Can you work these out from the model? Positions are in its coordinate system, mm. Face numbers are marked on the shaded views. A direction names the side the tool comes from. Round coordinates to 2 decimals unless told otherwise and drop trailing zeros. Order: outer loops, then holes, each group sorted by start corner. A loop starts at its lowest first (then second) coordinate and runs counter-clockwise, first axis right, second up. Notation, with made-up numbers: (32.5, 17) -> (68.5, 17) arc R28 cw to (68.5, 52) -> close; hole circle Ø3 at (-33, -31). An arc over 180 degrees is marked (long way). One line per item, written item: value.
```python
from build123d import *

# Parameters (mm, degrees)
F1_DEPTH = 25.4
F2_R     = 1.27
F3_R     = 2.286
F4_DEPTH = 7.62


with BuildPart() as f1:
    # F0 (on Top) → F1 (new body)
    with BuildSketch(Plane.XY):
        with BuildLine():
            Line((-44.880287, 2.54), (-3.81, 2.54))
            ThreePointArc((-3.81, 2.54), (-2.911974, 2.911974), (-2.54, 3.81))
            Line((-2.54, 3.81), (-2.54, 10.16))
            Line((-2.54, 10.16), (-15.24, 10.16))
            Line((-15.24, 10.16), (-15.24, 48.768))
            Line((-15.24, 48.768), (-32.180287, 48.768))
            ThreePointArc((-32.180287, 48.768), (-32.40082, 48.748706), (-32.614652, 48.69141))
            Line((-32.614652, 48.69141), (-52.504366, 41.452146))
            ThreePointArc((-52.504366, 41.452146), (-53.110323, 40.987179), (-53.34, 40.258736))
            Line((-53.34, 40.258736), (-53.34, 39.878))
            ThreePointArc((-53.34, 39.878), (-52.968026, 38.979974), (-52.07, 38.608))
            Line((-52.07, 38.608), (-29.21, 38.608))
            ThreePointArc((-29.21, 38.608), (-28.311974, 38.236026), (-27.94, 37.338))
            Line((-27.94, 37.338), (-27.94, 13.97))
            ThreePointArc((-27.94, 13.97), (-28.311974, 13.071974), (-29.21, 12.7))
            Line((-29.21, 12.7), (-64.77, 12.7))
            ThreePointArc((-64.77, 12.7), (-65.668026, 12.328026), (-66.04, 11.43))
            Line((-66.04, 11.43), (-66.04, 11.049264))
            ThreePointArc((-66.04, 11.049264), (-65.810323, 10.320821), (-65.204366, 9.855854))
            Line((-65.204366, 9.855854), (-45.314652, 2.61659))
            ThreePointArc((-45.314652, 2.61659), (-45.10082, 2.559294), (-44.880287, 2.54))
        make_face()
    extrude(amount=F1_DEPTH)

    # F2
    f2_edges = [f1.edges().sort_by_distance(p)[0] for p in [
        (-15.24, 10.16, 12.7),
        (-2.54, 10.16, 12.7),
        (-15.24, 48.768, 12.7),
    ]]
    fillet(f2_edges, radius=F2_R)

    # F3 (on face) → F4 (cut, through all)
    with BuildSketch(Plane(origin=(0, 10.16, 0), x_dir=(-1, 0, 0), z_dir=(0, 1, 0))):
        with Locations((8.89, 12.7)):
            Circle(F3_R)
    extrude(amount=-F4_DEPTH, mode=Mode.SUBTRACT)


solid = f1.part
```
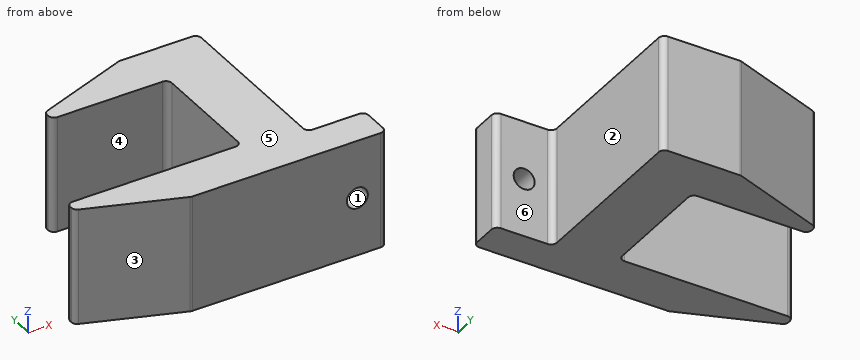
Q1. We'd pull the mould along X, two halves only. Please class the marked faces 1, 2 and 3: released by +X, released by -X, zero draft, split by the parting line, or undercut.
Answers below:
face 1: undercut
face 2: released by +X
face 3: released by -X
Q2. I want a section at D-D on x = -8.89. List the corners of the cut face in (y, z) for me.
Answers below:
outline: (2.54, 0) -> (10.16, 0) -> (10.16, 10.41) -> (2.54, 10.41) -> close; (2.54, 14.99) -> (10.16, 14.99) -> (10.16, 25.4) -> (2.54, 25.4) -> close
Q3. I want a section at C-C on z = 8.75. List the corners of the cut face in (x, y) for me, plus the area to 3 significant figures.
Answers below:
outline: (-66.04, 11.05) arc R1.27 ccw to (-65.2, 9.86) -> (-45.31, 2.62) arc R1.27 ccw to (-44.88, 2.54) -> (-3.81, 2.54) arc R1.27 ccw to (-2.54, 3.81) -> (-2.54, 8.89) arc R1.27 ccw to (-3.81, 10.16) -> (-13.97, 10.16) arc R1.27 cw to (-15.24, 11.43) -> (-15.24, 47.5) arc R1.27 ccw to (-16.51, 48.77) -> (-32.18, 48.77) arc R1.27 ccw to (-32.61, 48.69) -> (-52.5, 41.45) arc R1.27 ccw to (-53.34, 40.26) -> (-53.34, 39.88) arc R1.27 ccw to (-52.07, 38.61) -> (-29.21, 38.61) arc R1.27 cw to (-27.94, 37.34) -> (-27.94, 13.97) arc R1.27 cw to (-29.21, 12.7) -> (-64.77, 12.7) arc R1.27 ccw to (-66.04, 11.43) -> close
area: 1,170 mm^2
Q4. On a 3-axis mill with a long thin cutter (end or side, diameter ignored), from which of +Z, -Z, +X, -X, +Y, -Y can I reach the whole of each face in a straight line? I mean the marked faces 4, 5 and 6. Say none if no direction works.
Answers below:
face 4: +Z, -Z, -X
face 5: +Z, +X, -X, +Y, -Y
face 6: +Z, -Z, +X, +Y
Q5. Please list where these lines run through material, in increasing order: line 1 along Z through (x, y) = (-8.89, 8.25); line 2 along Y through (x, z) = (-30, 7); line 3 along X through (y, z) = (17.5, 1.5).
Answers below:
line 1: 0 to 10.41, 14.99 to 25.4
line 2: 2.54 to 12.7, 38.61 to 48.77
line 3: -27.94 to -15.24
Q6. I want a section at A-A on z = 12.7. List the corners of the cut face in (x, y) for me, plus the area to 3 significant figures.
Answers below:
outline: (-66.04, 11.05) arc R1.27 ccw to (-65.2, 9.86) -> (-45.31, 2.62) arc R1.27 ccw to (-44.88, 2.54) -> (-11.18, 2.54) -> (-11.18, 10.16) -> (-13.97, 10.16) arc R1.27 cw to (-15.24, 11.43) -> (-15.24, 47.5) arc R1.27 ccw to (-16.51, 48.77) -> (-32.18, 48.77) arc R1.27 ccw to (-32.61, 48.69) -> (-52.5, 41.45) arc R1.27 ccw to (-53.34, 40.26) -> (-53.34, 39.88) arc R1.27 ccw to (-52.07, 38.61) -> (-29.21, 38.61) arc R1.27 cw to (-27.94, 37.34) -> (-27.94, 13.97) arc R1.27 cw to (-29.21, 12.7) -> (-64.77, 12.7) arc R1.27 ccw to (-66.04, 11.43) -> close; (-6.6, 2.54) -> (-3.81, 2.54) arc R1.27 ccw to (-2.54, 3.81) -> (-2.54, 8.89) arc R1.27 ccw to (-3.81, 10.16) -> (-6.6, 10.16) -> close
area: 1,130 mm^2
Q7. I want a section at B-B on x = -31. List the corners of the cut face in (y, z) for me.
Answers below:
outline: (2.54, 0) -> (12.7, 0) -> (12.7, 25.4) -> (2.54, 25.4) -> close; (38.61, 0) -> (48.77, 0) -> (48.77, 25.4) -> (38.61, 25.4) -> close
Q8. Will these pins go through, and if not, where does the flat tip stop? pin 1 Ø7.5 at (x, z) = (-8.89, 12.7) entering from +Y; pin 2 Ø1.5 at (x, y) = (-13, 41) entering from -Z; pin 3 Ø10 at (x, z) = (-46.5, 8.5) entering from +Y; pin 4 Ø4 at (y, z) = (43.5, 17) entering from +X.
Answers below:
pin 1: y = 10.16
pin 2: through
pin 3: y = 45.46
pin 4: x = -15.24
